```python
from build123d import *

# Parameters (mm, degrees)
BOX002_W     = 3
BOX002_H     = 3
BOX002_DEPTH = 3
BOX003_W     = 3
BOX003_H     = 3
BOX003_DEPTH = 3
BOX004_W     = 3
BOX004_H     = 3
BOX004_DEPTH = 3
BOX005_W     = 3
BOX005_H     = 3
BOX005_DEPTH = 3
BOX001_W     = 10
BOX001_H     = 10
BOX001_DEPTH = 25
BOX012_W     = 3
BOX012_H     = 3
BOX012_DEPTH = 3
BOX013_W     = 3
BOX013_H     = 3
BOX013_DEPTH = 3
BOX014_W     = 3
BOX014_H     = 3
BOX014_DEPTH = 3
BOX015_W     = 3
BOX015_H     = 3
BOX015_DEPTH = 3
BOX011_W     = 10
BOX011_H     = 10
BOX011_DEPTH = 25
BOX017_W     = 3
BOX017_H     = 3
BOX017_DEPTH = 3
BOX018_W     = 3
BOX018_H     = 3
BOX018_DEPTH = 3
BOX019_W     = 3
BOX019_H     = 3
BOX019_DEPTH = 3
BOX020_W     = 3
BOX020_H     = 3
BOX020_DEPTH = 3
BOX016_W     = 10
BOX016_H     = 10
BOX016_DEPTH = 25
BOX021_W     = 50
BOX021_H     = 4
BOX021_DEPTH = 15
BOX022_W     = 50
BOX022_H     = 4
BOX022_DEPTH = 15
BOX023_W     = 50
BOX023_H     = 4
BOX023_DEPTH = 15
BOX024_W     = 10
BOX024_H     = 10
BOX024_DEPTH = 10
BOX_W        = 50
BOX_H        = 4
BOX_DEPTH    = 15
BOX007_W     = 3
BOX007_H     = 3
BOX007_DEPTH = 3
BOX008_W     = 3
BOX008_H     = 3
BOX008_DEPTH = 3
BOX009_W     = 3
BOX009_H     = 3
BOX009_DEPTH = 3
BOX010_W     = 3
BOX010_H     = 3
BOX010_DEPTH = 3
BOX006_W     = 10
BOX006_H     = 10
BOX006_DEPTH = 25


with BuildPart() as cubo001:
    # Box002 → Box002 (new body)
    with BuildSketch(Plane.XY.offset(25)):
        with Locations((1.5, 1.5)):
            Rectangle(BOX002_W, BOX002_H)
    extrude(amount=BOX002_DEPTH)


with BuildPart() as cubo002:
    # Box003 → Box003 (new body)
    with BuildSketch(Plane(origin=(7, 0, 25), x_dir=(1, 0, 0), z_dir=(0, 0, 1))):
        with Locations((1.5, 1.5)):
            Rectangle(BOX003_W, BOX003_H)
    extrude(amount=BOX003_DEPTH)


with BuildPart() as cubo003:
    # Box004 → Box004 (new body)
    with BuildSketch(Plane(origin=(7, 7, 25), x_dir=(1, 0, 0), z_dir=(0, 0, 1))):
        with Locations((1.5, 1.5)):
            Rectangle(BOX004_W, BOX004_H)
    extrude(amount=BOX004_DEPTH)


with BuildPart() as cubo004:
    # Box005 → Box005 (new body)
    with BuildSketch(Plane(origin=(0, 7, 25), x_dir=(1, 0, 0), z_dir=(0, 0, 1))):
        with Locations((1.5, 1.5)):
            Rectangle(BOX005_W, BOX005_H)
    extrude(amount=BOX005_DEPTH)


with BuildPart() as fusion:
    # Box001 → Box001 (new body)
    with BuildSketch(Plane.XY):
        with Locations((5, 5)):
            Rectangle(BOX001_W, BOX001_H)
    extrude(amount=BOX001_DEPTH)

    # Fusion: union Cubo001, Cubo002, Cubo003, Cubo004
    add(cubo001.part)
    add(cubo002.part)
    add(cubo003.part)
    add(cubo004.part)


with BuildPart() as cubo011:
    # Box012 → Box012 (new body)
    with BuildSketch(Plane.XY.offset(25)):
        with Locations((1.5, 1.5)):
            Rectangle(BOX012_W, BOX012_H)
    extrude(amount=BOX012_DEPTH)


with BuildPart() as cubo012:
    # Box013 → Box013 (new body)
    with BuildSketch(Plane(origin=(7, 0, 25), x_dir=(1, 0, 0), z_dir=(0, 0, 1))):
        with Locations((1.5, 1.5)):
            Rectangle(BOX013_W, BOX013_H)
    extrude(amount=BOX013_DEPTH)


with BuildPart() as cubo013:
    # Box014 → Box014 (new body)
    with BuildSketch(Plane(origin=(7, 7, 25), x_dir=(1, 0, 0), z_dir=(0, 0, 1))):
        with Locations((1.5, 1.5)):
            Rectangle(BOX014_W, BOX014_H)
    extrude(amount=BOX014_DEPTH)


with BuildPart() as cubo014:
    # Box015 → Box015 (new body)
    with BuildSketch(Plane(origin=(0, 7, 25), x_dir=(1, 0, 0), z_dir=(0, 0, 1))):
        with Locations((1.5, 1.5)):
            Rectangle(BOX015_W, BOX015_H)
    extrude(amount=BOX015_DEPTH)


with BuildPart() as fusion002:
    # Box011 → Box011 (new body)
    with BuildSketch(Plane.XY):
        with Locations((5, 5)):
            Rectangle(BOX011_W, BOX011_H)
    extrude(amount=BOX011_DEPTH)

    # Fusion002: union Cubo011, Cubo012, Cubo013, Cubo014
    add(cubo011.part)
    add(cubo012.part)
    add(cubo013.part)
    add(cubo014.part)


with BuildPart() as fusion002_1:
    # Fusion002 placement: moved
    add(fusion002.part.moved(Location((40, 40, 0))))


with BuildPart() as cubo016:
    # Box017 → Box017 (new body)
    with BuildSketch(Plane.XY.offset(25)):
        with Locations((1.5, 1.5)):
            Rectangle(BOX017_W, BOX017_H)
    extrude(amount=BOX017_DEPTH)


with BuildPart() as cubo017:
    # Box018 → Box018 (new body)
    with BuildSketch(Plane(origin=(7, 0, 25), x_dir=(1, 0, 0), z_dir=(0, 0, 1))):
        with Locations((1.5, 1.5)):
            Rectangle(BOX018_W, BOX018_H)
    extrude(amount=BOX018_DEPTH)


with BuildPart() as cubo018:
    # Box019 → Box019 (new body)
    with BuildSketch(Plane(origin=(7, 7, 25), x_dir=(1, 0, 0), z_dir=(0, 0, 1))):
        with Locations((1.5, 1.5)):
            Rectangle(BOX019_W, BOX019_H)
    extrude(amount=BOX019_DEPTH)


with BuildPart() as cubo019:
    # Box020 → Box020 (new body)
    with BuildSketch(Plane(origin=(0, 7, 25), x_dir=(1, 0, 0), z_dir=(0, 0, 1))):
        with Locations((1.5, 1.5)):
            Rectangle(BOX020_W, BOX020_H)
    extrude(amount=BOX020_DEPTH)


with BuildPart() as fusion003:
    # Box016 → Box016 (new body)
    with BuildSketch(Plane.XY):
        with Locations((5, 5)):
            Rectangle(BOX016_W, BOX016_H)
    extrude(amount=BOX016_DEPTH)

    # Fusion003: union Cubo016, Cubo017, Cubo018, Cubo019
    add(cubo016.part)
    add(cubo017.part)
    add(cubo018.part)
    add(cubo019.part)


with BuildPart() as fusion003_1:
    # Fusion003 placement: moved
    add(fusion003.part.moved(Location((0, 40, 0))))


with BuildPart() as wall001:
    # Box021 → Box021 (new body)
    with BuildSketch(Plane(origin=(0, 43, 0), x_dir=(1, 0, 0), z_dir=(0, 0, 1))):
        with Locations((25, 2)):
            Rectangle(BOX021_W, BOX021_H)
    extrude(amount=BOX021_DEPTH)


with BuildPart() as wall002:
    # Box022 → Box022 (new body)
    with BuildSketch(Plane(origin=(7, 0, 0), x_dir=(0, 1, 0), z_dir=(0, 0, 1))):
        with Locations((25, 2)):
            Rectangle(BOX022_W, BOX022_H)
    extrude(amount=BOX022_DEPTH)


with BuildPart() as wall003:
    # Box023 → Box023 (new body)
    with BuildSketch(Plane(origin=(47, 0, 0), x_dir=(0, 1, 0), z_dir=(0, 0, 1))):
        with Locations((25, 2)):
            Rectangle(BOX023_W, BOX023_H)
    extrude(amount=BOX023_DEPTH)


with BuildPart() as cubo020:
    # Box024 → Box024 (new body)
    with BuildSketch(Plane(origin=(20, 0, 0), x_dir=(1, 0, 0), z_dir=(0, 0, 1))):
        with Locations((5, 5)):
            Rectangle(BOX024_W, BOX024_H)
    extrude(amount=BOX024_DEPTH)


with BuildPart() as cut:
    # Box → Box (new body)
    with BuildSketch(Plane(origin=(0, 3, 0), x_dir=(1, 0, 0), z_dir=(0, 0, 1))):
        with Locations((25, 2)):
            Rectangle(BOX_W, BOX_H)
    extrude(amount=BOX_DEPTH)

    # Cut: cut Cubo020
    add(cubo020.part, mode=Mode.SUBTRACT)


with BuildPart() as cubo006:
    # Box007 → Box007 (new body)
    with BuildSketch(Plane.XY.offset(25)):
        with Locations((1.5, 1.5)):
            Rectangle(BOX007_W, BOX007_H)
    extrude(amount=BOX007_DEPTH)


with BuildPart() as cubo007:
    # Box008 → Box008 (new body)
    with BuildSketch(Plane(origin=(7, 0, 25), x_dir=(1, 0, 0), z_dir=(0, 0, 1))):
        with Locations((1.5, 1.5)):
            Rectangle(BOX008_W, BOX008_H)
    extrude(amount=BOX008_DEPTH)


with BuildPart() as cubo008:
    # Box009 → Box009 (new body)
    with BuildSketch(Plane(origin=(7, 7, 25), x_dir=(1, 0, 0), z_dir=(0, 0, 1))):
        with Locations((1.5, 1.5)):
            Rectangle(BOX009_W, BOX009_H)
    extrude(amount=BOX009_DEPTH)


with BuildPart() as cubo009:
    # Box010 → Box010 (new body)
    with BuildSketch(Plane(origin=(0, 7, 25), x_dir=(1, 0, 0), z_dir=(0, 0, 1))):
        with Locations((1.5, 1.5)):
            Rectangle(BOX010_W, BOX010_H)
    extrude(amount=BOX010_DEPTH)


with BuildPart() as fusion004:
    # Box006 → Box006 (new body)
    with BuildSketch(Plane.XY):
        with Locations((5, 5)):
            Rectangle(BOX006_W, BOX006_H)
    extrude(amount=BOX006_DEPTH)

    # Fusion001: union Cubo006, Cubo007, Cubo008, Cubo009
    add(cubo006.part)
    add(cubo007.part)
    add(cubo008.part)
    add(cubo009.part)


with BuildPart() as fusion004_1:
    # Fusion001 placement: moved
    add(fusion004.part.moved(Location((40, 0, 0))))

    # Fusion004: union Fusion, Fusion002, Fusion003, wall001, wall002, wall003, Cut
    add(fusion.part)
    add(fusion002_1.part)
    add(fusion003_1.part)
    add(wall001.part)
    add(wall002.part)
    add(wall003.part)
    add(cut.part)


solid = fusion004_1.part
```
Design review of the part built by this model. Coordinates are the model's own, in mm. A direction names the side the tool comes from. Coordinates: 2 decimals unless noted, no trailing zeros. Order: outer loops, then holes, each group sorted by start corner. A loop starts at its lowest first (then second) coordinate and runs counter-clockwise, first axis right, second up. Notation, with made-up numbers: (-11.5, -17.5) - (36.5, -17.5) arc R3 cw to (36.5, -13.5) - close; hole circle Ø7 at (42.5, -20). An arc over 180 degrees is marked (long way). Answer in a Markdown table with one row per item.
(1) Consider section D-D on y = 45.5. State the section outline as (x, z) points.
Checked values:
| item | result |
|---|---|
| outline | (0, 0) - (50, 0) - (50, 25) - (40, 25) - (40, 15) - (10, 15) - (10, 25) - (0, 25) - close |
(2) Wall thickness on line 1 along Y through (x, z) = (48.5, 27); line 2 along Y through (x, z) = (45, 21.5): over which ranges is each line inside the solid? List them lowest first. Write a range as from..to.
Checked values:
| item | result |
|---|---|
| line 1 | 0..3, 7..10, 40..43, 47..50 |
| line 2 | 0..10, 40..50 |
(3) For faces 1 (the flat face through (25, 47, 7)), 2 (the flat face through (20, 5, 5)), 3 (the flat face through (41, 3, 26)), 4 (the flat face through (5, 40, 17)), list the 3-axis set-ups (+Z, -Z, +X, -X, +Y, -Y) from which the entire face can be reached by the end or side of a thin tool; tool diameter is ignored.
Checked values:
| item | result |
|---|---|
| face 1 | +Z, -Z, +Y |
| face 2 | -Z, -Y |
| face 3 | +Z, +X, -X |
| face 4 | +Z |
(4) Clearance check with flat-ended pins moving along their axes: pin 1 (12 mm diameter, centred on y = 17, z = 19.5, fed in from -X); pin 2 (12 mm diameter, centred on y = 26.5, z = 8, fed in from +X); pin 3 (1.5 mm diameter, centred on x = 24, z = 6, fed in from +Y). State where each tip first meets the part, or that it passes through.
Checked values:
| item | result |
|---|---|
| pin 1 | x = 3 |
| pin 2 | x = 47 |
| pin 3 | y = 47 |
(5) The part is to be moulded in two halves that separate along X. For faces 5 (the flat face through (3, 8, 26)), 6 (the flat face through (8, 3, 26)), 7 (the flat face through (40, 5, 17)), say which applies: released by +X, released by -X, zero draft, split by the parting line, or undercut.
Checked values:
| item | result |
|---|---|
| face 5 | undercut |
| face 6 | zero draft |
| face 7 | undercut |
(6) Consider section A-A on x = 25.5. State the section outline as (y, z) points, plus the area to 3 significant figures.
Checked values:
| item | result |
|---|---|
| outline | (3, 10) - (7, 10) - (7, 15) - (3, 15) - close; (43, 0) - (47, 0) - (47, 15) - (43, 15) - close |
| area | 80.0 mm^2 |
(7) Consider section C-C on z = 22. State the section outline as (x, y) points, plus the area to 3 significant figures.
Checked values:
| item | result |
|---|---|
| outline | (0, 0) - (10, 0) - (10, 10) - (0, 10) - close; (0, 40) - (10, 40) - (10, 50) - (0, 50) - close; (40, 0) - (50, 0) - (50, 10) - (40, 10) - close; (40, 40) - (50, 40) - (50, 50) - (40, 50) - close |
| area | 400 mm^2 |
(8) Consider section B-B on y = 27. State the section outline as (x, z) points, plus the area to 3 significant figures.
Checked values:
| item | result |
|---|---|
| outline | (3, 0) - (7, 0) - (7, 15) - (3, 15) - close; (43, 0) - (47, 0) - (47, 15) - (43, 15) - close |
| area | 120 mm^2 |
